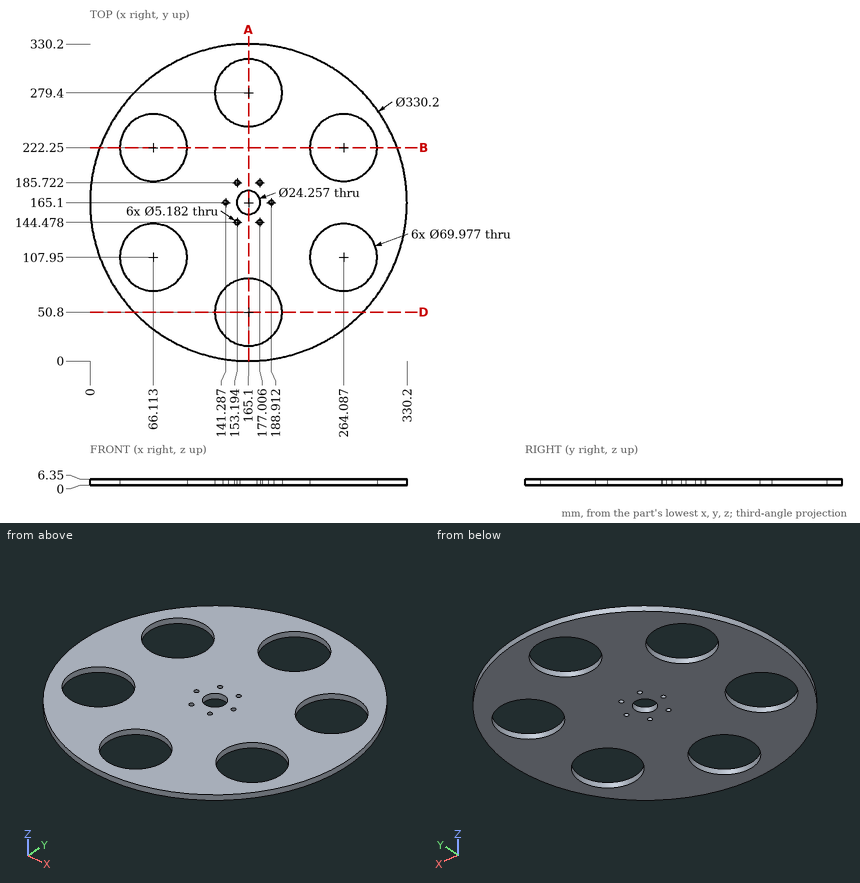
Study the drawing (mm; zero at the part's minimum x, y, z) and answer. Round coordinates to 2 decimals unless told otherwise and drop trailing zeros. Write each loop counter-clockwise with the first axis right and the second up, starting at its lowest first coordinate (ties: lowest second). Pieces come first, ordered by that corner, then holes. Notation, with made-up numbers: (72, 84) - (115, 84) arc R8 cw to (115, 90) - close; hole circle Ø8 at (47, -35). An arc over 180 degrees is marked (long way). Use a Markdown table: item, result. Add a question column.
1. The part is cut by section B-B (y = 222.25). Give the number of separate pieces and of enclosed holes in the cut face, and give its area (3 significant figures).
2. The part is cut by section D-D (y = 50.8). Write down the section's boundary in (x, z).
3. Flat-ended cylindrical pins translate along their axes: P1, Ø1.5, axis at y = 55, z = 3, coming from the +X side (1 decimal); P2, Ø2, axis at x = 66.5, z = 3.5, coming from the -Y side; P3, Ø3, axis at x = 141.29, y = 165.1, coming from the +Z side. Find the tip coordinate at first contact, or state that the pin passes through.
4. Consider line 1 (Y direction, x = 165.1, z = 1.5); line 2 (X direction, y = 163, z = 0.5) (1 decimal); line 3 (Y direction, x = 247, z = 4) (1 decimal). Determine where each line is inside the solid, lowest interval first.
5. The part is cut by section A-A (x = 165.1). Write down the section's boundary in (y, z).
Reported:
| question | item | result |
|---|---|---|
| 1 | separate pieces | 3 |
| 1 | enclosed holes | 0 |
| 1 | area | 1,080 mm^2 |
| 2 | outline | (45.96, 0) - (130.11, 0) - (130.11, 6.35) - (45.96, 6.35) - close; (200.09, 0) - (284.24, 0) - (284.24, 6.35) - (200.09, 6.35) - close |
| 3 | P1 | x = 288.8 |
| 3 | P2 | y = 31.94 |
| 3 | P3 | through |
| 4 | line 1 | 0 to 15.81, 85.79 to 152.97, 177.23 to 244.41, 314.39 to 330.2 |
| 4 | line 2 | 0 to 139.8, 142.8 to 153.2, 177 to 187.4, 190.4 to 330.2 |
| 4 | line 3 | 21.7 to 77.4, 138.5 to 191.7, 252.8 to 308.5 |
| 5 | outline | (0, 0) - (15.81, 0) - (15.81, 6.35) - (0, 6.35) - close; (85.79, 0) - (152.97, 0) - (152.97, 6.35) - (85.79, 6.35) - close; (177.23, 0) - (244.41, 0) - (244.41, 6.35) - (177.23, 6.35) - close; (314.39, 0) - (330.2, 0) - (330.2, 6.35) - (314.39, 6.35) - close |
